from build123d import *

# Parameters (mm, degrees)
SKETCH_1_W          = 4.5
SKETCH_1_H          = 41
EXTRUDE_1_DEPTH     = 8
SKETCH_3_W          = 2
SKETCH_3_H          = 41
CUT_EXTRUDE_1_DEPTH = 7
SKETCH_5_R          = 2.5
CUT_EXTRUDE_2_DEPTH = 23.461077445
FILLET_1_R          = 3


with BuildPart() as part:
    # Эскиз1 → Бобышка-Вытянуть1 (new body)
    with BuildSketch(Plane.XY):
        Rectangle(SKETCH_1_W, SKETCH_1_H)
    extrude(amount=EXTRUDE_1_DEPTH)

    # Эскиз3 → Вырез-Вытянуть1 (cut)
    with BuildSketch(Plane.XY.offset(8)):
        with Locations((0.25, 0)):
            Rectangle(SKETCH_3_W, SKETCH_3_H)
    extrude(amount=-CUT_EXTRUDE_1_DEPTH, mode=Mode.SUBTRACT)

    # Эскиз5 → Вырез-Вытянуть2 (cut, through all)
    with BuildSketch(Plane(origin=(2.25, 0, 0), x_dir=(0, 0, -1), z_dir=(1, 0, 0))):
        with Locations(Location((-4, 14, 0), (0, 0, 90))):
            Circle(SKETCH_5_R)
        with Locations(Location((-4, -15.5, 0), (0, 0, 90))):
            Circle(SKETCH_5_R)
    extrude(amount=-CUT_EXTRUDE_2_DEPTH, mode=Mode.SUBTRACT)

    # Скругление1
    fillet_1_edges = [part.edges().sort_by_distance(p)[0] for p in [
        (-1.5, 20.5, 8),
        (1.75, -20.5, 8),
        (-1.5, -20.5, 8),
        (1.75, 20.5, 8),
    ]]
    fillet(fillet_1_edges, radius=FILLET_1_R)


solid = part.part
Here's how the part is built. I have some questions about the finished solid (model axes, mm). A direction names the side the tool comes from. Give positions to 0.01 mm unless a question says otherwise; leave off trailing zeros. Order: outer loops, then holes, each group sorted by start corner. A loop starts at its lowest first (then second) coordinate and runs counter-clockwise, first axis right, second up. Notation, with made-up numbers: (51.25, 62.25) -> (77.25, 62.25) arc R27 ccw to (77.25, 96.25) -> close; hole circle Ø6 at (-10, -37.75). An arc over 180 degrees is marked (long way). Use a Markdown table: item, result. Add a question column.
Item 1: Imagine slicing it at C-C on x = -1.5. Please give me the cut outline in (y, z).
Item 2: Imagine slicing it at D-D on y = 2.5. Please give me the cut outline in (x, z).
Item 3: Imagine slicing it at A-A on y = 14. Please give me the cut outline in (x, z), plus the area to 3 significant figures.
Item 4: If we mould it in two halves opening along X, with no side actions, what happens to faces 3 (the face through (-1, -18, 4)), 4 (the face through (-2.25, 0, 4)), 5 (the face through (0, 0, 1))? For each: pulls with the +X half, pulls with the -X half, needs draft (parallel to the pull), parting line crosses it, or undercut.
Item 5: For faces 1 (the face through (-2, 0, 8)), 2 (the face through (1.25, 0, 5)), which set-ups out of +Z, -Z, +X, -X, +Y, -Y let a thin tool reach every point of the face, with its end or its side?
Item 6: I need wall thicknesses on line 1 (X direction, y = -11.5, z = 2); line 2 (Z direction, x = 1.9, y = -15.5); line 3 (Y direction, x = -1.9, z = 1.75). Which ranges of each line are inside material? Lowest first, please.
Item 7: Will these pins go through, and if not, where does the flat tip stop? pin 1 (0.6 mm diameter, centred on x = 0.5, y = 5, fed in from +Z); pin 2 (1.5 mm diameter, centred on x = -1.5, z = 6, fed in from +Y).
Item 8: Imagine slicing it at B-B on z = 4. Please give me the cut outline in (x, y), plus the area to 3 significant figures.
Data:
| question | item | result |
|---|---|---|
| 1 | outline | (-20.5, 0) -> (20.5, 0) -> (20.5, 5) arc R3 ccw to (17.5, 8) -> (-17.5, 8) arc R3 ccw to (-20.5, 5) -> close; hole circle Ø5 at (-15.5, 4); hole circle Ø5 at (14, 4) |
| 2 | outline | (-2.25, 0) -> (2.25, 0) -> (2.25, 8) -> (1.25, 8) -> (1.25, 1) -> (-0.75, 1) -> (-0.75, 8) -> (-2.25, 8) -> close |
| 3 | outline | (-2.25, 0) -> (2.25, 0) -> (2.25, 1.5) -> (1.25, 1.5) -> (1.25, 1) -> (-0.75, 1) -> (-0.75, 1.5) -> (-2.25, 1.5) -> close; (-2.25, 6.5) -> (-0.75, 6.5) -> (-0.75, 8) -> (-2.25, 8) -> close; (1.25, 6.5) -> (2.25, 6.5) -> (2.25, 8) -> (1.25, 8) -> close |
| 3 | area | 9.50 mm² |
| 4 | face 3 | needs draft |
| 4 | face 4 | pulls with the -X half |
| 4 | face 5 | undercut |
| 5 | face 1 | +Z, +X, -X, +Y, -Y |
| 5 | face 2 | +Z, +Y, -Y |
| 6 | line 1 | x = -2.25 to -0.75, 1.25 to 2.25 |
| 6 | line 2 | z = 0 to 1.5, 6.5 to 8 |
| 6 | line 3 | y = -20.5 to -16.59, -14.41 to 12.91, 15.09 to 20.5 |
| 7 | pin 1 | stops at z = 1 |
| 7 | pin 2 | stops at y = 20.49 |
| 8 | outline | (-2.25, -20.5) -> (-0.75, -20.5) -> (-0.75, -18) -> (-2.25, -18) -> close; (-2.25, -13) -> (-0.75, -13) -> (-0.75, 11.5) -> (-2.25, 11.5) -> close; (-2.25, 16.5) -> (-0.75, 16.5) -> (-0.75, 20.5) -> (-2.25, 20.5) -> close; (1.25, -20.5) -> (2.25, -20.5) -> (2.25, -18) -> (1.25, -18) -> close; (1.25, -13) -> (2.25, -13) -> (2.25, 11.5) -> (1.25, 11.5) -> close; (1.25, 16.5) -> (2.25, 16.5) -> (2.25, 20.5) -> (1.25, 20.5) -> close |
| 8 | area | 77.5 mm² |
